Work out the finished part from the listing and answer in its coordinate system (mm). Face numbers are marked on the shaded views. Give positions to 0.01 mm unless a question says otherwise; leave off trailing zeros. Order: outer loops, then holes, each group sorted by start corner. A loop starts at its lowest first (then second) coordinate and runs counter-clockwise, first axis right, second up.
```python
from build123d import *

# Parameters (mm, degrees)
ESQUISSE1_W        = 45
ESQUISSE1_H        = 10
ESQUISSE1_R        = 1.5
ESQUISSE1_R_2      = 2
BOSS_EXTRU_1_DEPTH = 6
CONG_1_R           = 2


with BuildPart() as part:
    # Esquisse1 → Boss.-Extru.1 (new body)
    with BuildSketch(Plane.XY):
        with Locations((22.5, 5)):
            Rectangle(ESQUISSE1_W, ESQUISSE1_H)
        with Locations((5, 5)):
            Circle(ESQUISSE1_R, mode=Mode.SUBTRACT)
        with Locations((22.5, 5)):
            Circle(ESQUISSE1_R_2, mode=Mode.SUBTRACT)
        with Locations((40, 5)):
            Circle(ESQUISSE1_R, mode=Mode.SUBTRACT)
    extrude(amount=BOSS_EXTRU_1_DEPTH)

    # Congé1
    cong_1_edges = [part.edges().sort_by_distance(p)[0] for p in [
        (22.5, 10, 0),
        (45, 5, 0),
        (22.5, 0, 0),
        (0, 5, 0),
    ]]
    fillet(cong_1_edges, radius=CONG_1_R)


solid = part.part
```
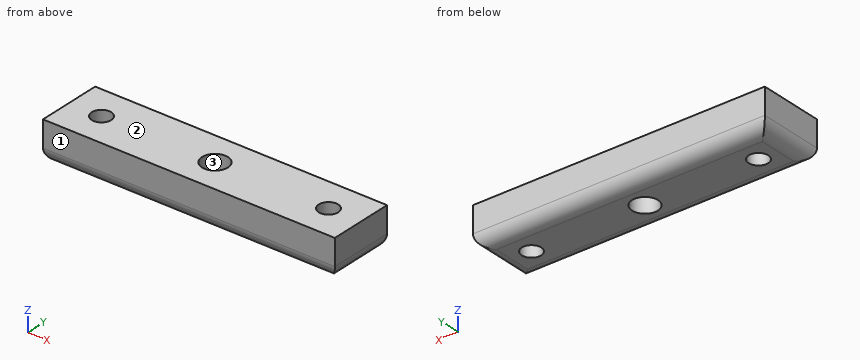
1. The part is cut by section D-D (x = 22.5). Write down the section's boundary in (y, z), then the cut area to 3 significant figures.
Findings below:
outline: (0, 2) arc R2 ccw to (2, 0) - (3, 0) - (3, 6) - (0, 6) - close; (7, 0) - (8, 0) arc R2 ccw to (10, 2) - (10, 6) - (7, 6) - close
area: 34.3 mm2
2. Given P1, Ø3, axis at x = 22.5, y = 5, coming from the +Z side, flat-ended and moving along its own axis, determine where the tip first touches the part or whether it passes through.
Findings below:
P1: passes through
3. The part is cut by section B-B (y = 5). Write down the section's boundary in (x, z).
Findings below:
outline: (0, 2) arc R2 ccw to (2, 0) - (3.5, 0) - (3.5, 6) - (0, 6) - close; (6.5, 0) - (20.5, 0) - (20.5, 6) - (6.5, 6) - close; (24.5, 0) - (38.5, 0) - (38.5, 6) - (24.5, 6) - close; (41.5, 0) - (43, 0) arc R2 ccw to (45, 2) - (45, 6) - (41.5, 6) - close
4. The part is cut by section A-A (x = 5). Write down the section's boundary in (y, z), then the cut area to 3 significant figures.
Findings below:
outline: (0, 2) arc R2 ccw to (2, 0) - (3.5, 0) - (3.5, 6) - (0, 6) - close; (6.5, 0) - (8, 0) arc R2 ccw to (10, 2) - (10, 6) - (6.5, 6) - close
area: 40.3 mm2
5. The mould has two halves that part along Y. Classify the marked faces 1, 2 and 3: pulls with the +Y half, pulls with the -Y half, needs draft (parallel to the pull), parting line crosses it, or undercut.
Findings below:
face 1: pulls with the -Y half
face 2: needs draft
face 3: undercut
6. The part is cut by section C-C (z = 2.6). Write down the section's boundary in (x, y), then the cut area to 3 significant figures.
Findings below:
outline: (0, 0) - (45, 0) - (45, 10) - (0, 10) - close; hole circle Ø3 at (5, 5); hole circle Ø4 at (22.5, 5); hole circle Ø3 at (40, 5)
area: 423 mm2
7. Straight lines are drawn through the part: probe 1 along Y at (x, z) = (40, 3.1); probe 2 along Y at (x, z) = (22.5, 3.2); probe 3 along X at (y, z) = (5.25, 5.8). For each, find the intervals that lie inside material, in ascending order.
Findings below:
probe 1: y = 0 to 3.5, 6.5 to 10
probe 2: y = 0 to 3, 7 to 10
probe 3: x = 0 to 3.52, 6.48 to 20.52, 24.48 to 38.52, 41.48 to 45
